Study the drawing (mm; zero at the part's minimum x, y, z) and answer. Give positions to 0.01 mm unless a question says otherwise; leave off trailing zeros. Write each loop counter-clockwise with the first axis right and the second up, starting at its lowest first coordinate (ties: lowest second). Pieces come first, ordered by that corner, then holes. Notation, with made-up numbers: (26.5, -1.75) - (68.5, -1.75) arc R23 ccw to (68.5, 9.25) - close; hole circle Ø2 at (27, 57). An arc over 180 degrees is marked (long way). Answer in a Markdown table with one row per item. Add a question column.
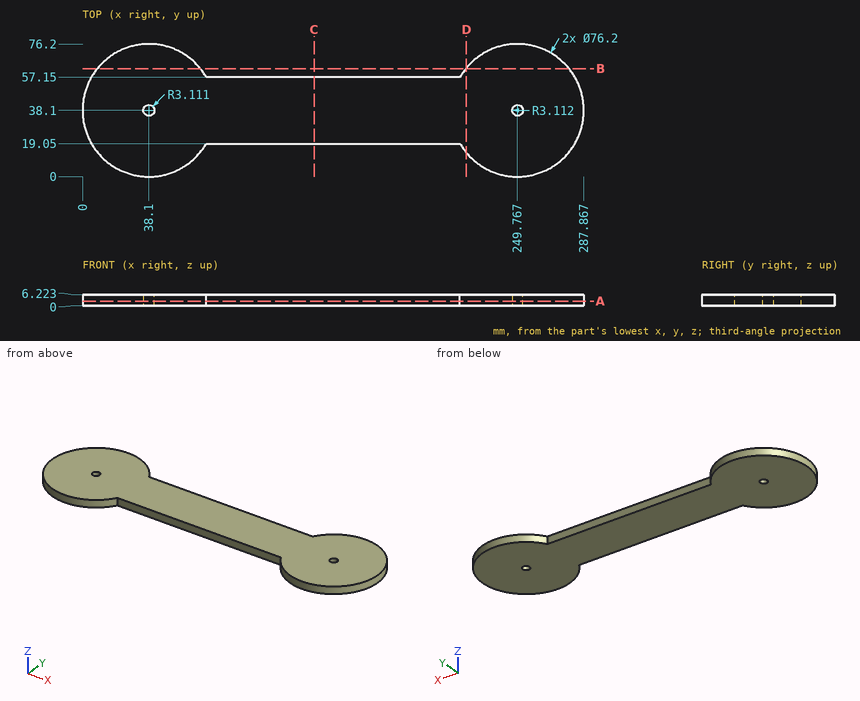
1. Section C-C (x = 133) is taken. Give the vertices of the cut face in (y, z).
2. Section B-B (y = 62) is taken. Give the vertices of the cut face in (x, z) (1 decimal).
3. Section D-D (x = 220.5) is taken. Give the vertices of the cut face in (y, z) (1 decimal).
4. Straight lines are drawn through the part: L1, parallel to X at y = 39, z = 0.5 (1 decimal); L2, parallel to Y at x = 114, z = 5.75; L3, parallel to X at y = 8, z = 3.5 (1 decimal). For each, find the intervals that lie inside material, in ascending order. Write a range as [from, to].
5. Given pin 1 Ø1.5 at (y, z) = (40.5, 2) entering from +X; pin 2 Ø2 at (x, z) = (172, 5) entering from -Y; pin 3 Ø2 at (x, z) = (94.5, 3) entering from +Y, each flat-ended and moving along its own axis, determine where each tip first touches the part or whether it passes through.
6. Section A-A (z = 2.5) is taken. State how many separate pieces and enclosed holes the cut face has, and give its area (3 significant figures).
Geometry check:
| question | item | result |
|---|---|---|
| 1 | outline | (19.05, 0) - (57.15, 0) - (57.15, 6.22) - (19.05, 6.22) - close |
| 2 | outline | (8.4, 0) - (67.8, 0) - (67.8, 6.2) - (8.4, 6.2) - close; (220.1, 0) - (279.4, 0) - (279.4, 6.2) - (220.1, 6.2) - close |
| 3 | outline | (13.7, 0) - (62.5, 0) - (62.5, 6.2) - (13.7, 6.2) - close |
| 4 | L1 | [0, 35.1], [41.1, 246.8], [252.7, 287.9] |
| 4 | L2 | [19.05, 57.15] |
| 4 | L3 | [14.7, 61.5], [226.4, 273.1] |
| 5 | pin 1 | x = 287.83 |
| 5 | pin 2 | y = 19.05 |
| 5 | pin 3 | y = 57.15 |
| 6 | separate pieces | 1 |
| 6 | enclosed holes | 2 |
| 6 | area | 14,300 mm² |
